```python
from build123d import *

# Parameters (mm, degrees)
F0_W          = 38
F0_H          = 23
F1_DEPTH      = 4.5
F2_T          = -2
F3_W          = 9
F3_H          = 2.5
F4_DEPTH      = 2
F5_W          = 2
F5_H          = 1
F6_DEPTH      = 2
F7_W          = 4
F7_H          = 4
F7_H_2        = 4.2236842105
F8_DEPTH      = 2
F9_DEPTH      = 0.5
F10_W         = 4
F10_H         = 4
F10_H_2       = 5.5396806626
F11_DEPTH     = 2
F12_DEPTH     = 0.5
F13_SIZE2     = 1
F13_SIZE      = 1
F14_T1_DEPTH  = 14.2867319519
F14_T3_DEPTH  = 14.2867319519
F14_T5_DEPTH  = 14.2867319519
F14_T10_DEPTH = 14.2867319519
F14_T15_DEPTH = 14.2867319519
F14_T20_DEPTH = 14.2867319519
F15_R         = 2
F10_H_3       = 1.5
F16_DEPTH     = 1
F7_H_3        = 1.5
F17_DEPTH     = 1
F18_SIZE2     = 0.99999
F18_SIZE      = 1.49999
F19_SIZE2     = 1.49999
F19_SIZE      = 0.99999
F20_SIZE2     = 0.99999
F20_SIZE      = 1.49999


# Not quite as in the source:
# - a fillet or chamfer that OpenCascade refuses, or shapes differently, is made with other operations: its cross-section is extruded or revolved along the edge and cut away or added
# - a fillet or chamfer is up to 0.001 mm smaller than in the source, because OpenCascade refuses the exact size


with BuildPart() as f1:
    # F0 (on Top) → F1 (new body)
    with BuildSketch(Plane.XY):
        Rectangle(F0_W, F0_H)
    extrude(amount=F1_DEPTH)

    # F2
    f2_openings = [f1.faces().sort_by_distance(p)[0] for p in [
        (0, 0, 4.5),
    ]]
    offset(amount=F2_T, openings=f2_openings)

    # F3 (on face) → F4 (cut, through all)
    with BuildSketch(Plane(origin=(-19, 0, 0), x_dir=(0, -1, 0), z_dir=(-1, 0, 0))):
        with Locations((0, 3.25)):
            Rectangle(F3_W, F3_H)
    extrude(amount=-F4_DEPTH, mode=Mode.SUBTRACT)

    # F5 (on face) → F6 (cut, through all)
    with BuildSketch(Plane(origin=(0, 11.5, 0), x_dir=(-1, 0, 0), z_dir=(0, 1, 0))):
        with Locations((-2.0402920675, 4)):
            Rectangle(F5_W, F5_H)
        with Locations((2.0402920675, 4)):
            Rectangle(F5_W, F5_H)
    extrude(amount=-F6_DEPTH, mode=Mode.SUBTRACT)

    # F7 (on face) → F8 (join)
    with BuildSketch(Plane(origin=(0, 11.5, 0), x_dir=(-1, 0, 0), z_dir=(0, 1, 0))):
        with Locations((-9.5, 8)):
            Rectangle(F7_W, F7_H)
        with Locations((-9.5, 3.8881578947)):
            Rectangle(F7_W, F7_H_2)
        with Locations((9.5, 8)):
            Rectangle(F7_W, F7_H)
        with Locations((9.5, 3.8881578947)):
            Rectangle(F7_W, F7_H_2)
    extrude(amount=F8_DEPTH)

    # F7 (on face) → F9 (join)
    with BuildSketch(Plane(origin=(0, 11.5, 0), x_dir=(-1, 0, 0), z_dir=(0, 1, 0))):
        with Locations((-9.5, 8)):
            Rectangle(F7_W, F7_H)
        with Locations((9.5, 8)):
            Rectangle(F7_W, F7_H)
    extrude(amount=-F9_DEPTH)

    # F10 (on face) → F11 (join)
    with BuildSketch(Plane.XZ.offset(11.5)):
        with Locations((0, 8)):
            Rectangle(F10_W, F10_H)
        with Locations((0, 3.2301596687)):
            Rectangle(F10_W, F10_H_2)
    extrude(amount=F11_DEPTH)

    # F10 (on face) → F12 (join)
    with BuildSketch(Plane.XZ.offset(11.5)):
        with Locations((0, 8)):
            Rectangle(F10_W, F10_H)
    extrude(amount=-F12_DEPTH)

    # F13
    f13_edges = [f1.edges().sort_by_distance(p)[0] for p in [
        (0, -11, 10),
        (-9.5, 11, 10),
        (9.5, 11, 10),
    ]]
    chamfer(f13_edges, length=F13_SIZE, length2=F13_SIZE2)

    # F14: chamfer of 2 on 6 edges, made by hand

    # F14_s2 → F14_t1 (cut)
    with BuildSketch(Plane.YZ.offset(2.3566340241)):
        Polygon((11.5, 10), (13.5, 8), (13.5, 10), align=None)
    extrude(amount=F14_T1_DEPTH, mode=Mode.SUBTRACT)

    # F14_s4 → F14_t3 (cut)
    with BuildSketch(Plane.YZ.offset(-16.6433659759)):
        Polygon((11.5, 10), (13.5, 8), (13.5, 10), align=None)
    extrude(amount=F14_T3_DEPTH, mode=Mode.SUBTRACT)

    # F14_s6 → F14_t5 (cut)
    with BuildSketch(Plane.YZ.offset(-7.1433659759)):
        Polygon((-11.5, 10), (-13.5, 8), (-13.5, 10), align=None)
    extrude(amount=F14_T5_DEPTH, mode=Mode.SUBTRACT)


with BuildPart() as f14_tool8:
    # F14_s9 → F14_t10 (new body)
    with BuildSketch(Plane.YZ.offset(-2.3566340241)):
        Polygon((11.5, 1.7763157895), (13.5, 3.7763157895), (13.5, 1.7763157895), align=None)
    extrude(amount=-F14_T10_DEPTH)

    split(bisect_by=Plane.XZ.offset(-11.5), keep=Keep.BOTTOM)


with BuildPart() as f1_1:
    add(f1.part)

    # F14_t7: cut F14_tool8
    add(f14_tool8.part, mode=Mode.SUBTRACT)


with BuildPart() as f14_tool13:
    # F14_s14 → F14_t15 (new body)
    with BuildSketch(Plane.YZ.offset(16.6433659759)):
        Polygon((13.5, 3.7763157895), (11.5, 1.7763157895), (13.5, 1.7763157895), align=None)
    extrude(amount=-F14_T15_DEPTH)

    split(bisect_by=Plane.XZ.offset(-11.5), keep=Keep.BOTTOM)


with BuildPart() as f1_2:
    add(f1_1.part)

    # F14_t12: cut F14_tool13
    add(f14_tool13.part, mode=Mode.SUBTRACT)


with BuildPart() as f14_tool18:
    # F14_s19 → F14_t20 (new body)
    with BuildSketch(Plane.YZ.offset(-7.1433659759)):
        Polygon((-11.5, 0.4603193374), (-13.5, 2.4603193374), (-13.5, 0.4603193374), align=None)
    extrude(amount=F14_T20_DEPTH)

    split(bisect_by=Plane.XZ.offset(11.5), keep=Keep.TOP)


with BuildPart() as f1_3:
    add(f1_2.part)

    # F14_t17: cut F14_tool18
    add(f14_tool18.part, mode=Mode.SUBTRACT)

    # F15
    f15_edges = [f1_3.edges().sort_by_distance(p)[0] for p in [
        (19, -11.5, 2.25),
        (19, 11.5, 2.25),
        (-19, 11.5, 2.25),
        (-19, -11.5, 2.25),
    ]]
    fillet(f15_edges, radius=F15_R)

    # F10 (on face) → F16 (cut)
    with BuildSketch(Plane.XZ.offset(11.5)):
        with Locations((0, 5.25)):
            Rectangle(F10_W, F10_H_3)
    extrude(amount=F16_DEPTH, mode=Mode.SUBTRACT)

    # F7 (on face) → F17 (cut)
    with BuildSketch(Plane(origin=(0, 11.5, 0), x_dir=(-1, 0, 0), z_dir=(0, 1, 0))):
        with Locations((9.5, 5.25)):
            Rectangle(F7_W, F7_H_3)
        with Locations((-9.5, 5.25)):
            Rectangle(F7_W, F7_H_3)
    extrude(amount=F17_DEPTH, mode=Mode.SUBTRACT)

    # F18 (size 1.5 and 1 in the source; OpenCascade refuses exactly that, so slightly less here)
    f18_edges = [f1_3.edges().sort_by_distance(p)[0] for p in [
        (0, -11, 6),
    ]]
    f18_side = f1_3.faces().sort_by_distance((0, -11.75, 6))[0]
    chamfer(f18_edges, length=F18_SIZE, length2=F18_SIZE2, reference=f18_side)

    # F19 (size 1 and 1.5 in the source; OpenCascade refuses exactly that, so slightly less here)
    f19_edges = [f1_3.edges().sort_by_distance(p)[0] for p in [
        (-9.5, 11, 6),
    ]]
    f19_side = f1_3.faces().sort_by_distance((-9.5, 11, 7.5))[0]
    chamfer(f19_edges, length=F19_SIZE, length2=F19_SIZE2, reference=f19_side)

    # F20 (size 1.5 and 1 in the source; OpenCascade refuses exactly that, so slightly less here)
    f20_edges = [f1_3.edges().sort_by_distance(p)[0] for p in [
        (9.5, 11, 6),
    ]]
    f20_side = f1_3.faces().sort_by_distance((9.5, 11.75, 6))[0]
    chamfer(f20_edges, length=F20_SIZE, length2=F20_SIZE2, reference=f20_side)


solid = f1_3.part
```
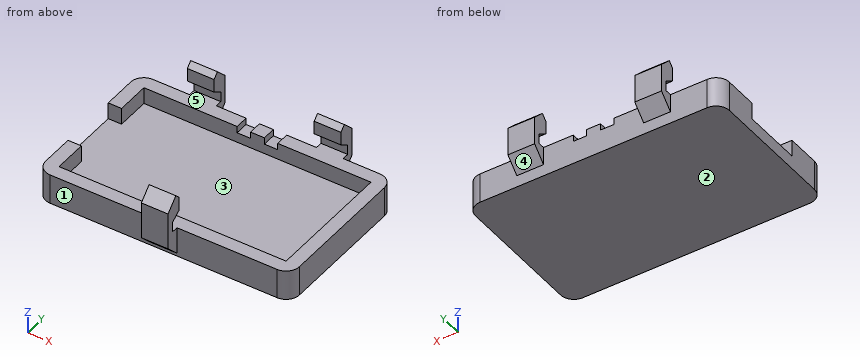
Here's how the part is built. I have some questions about the finished solid (model axes, mm). Face numbers are marked on the shaded views. A direction names the side the tool comes from. Coordinates: 2 decimals unless noted, no trailing zeros. Write each loop counter-clockwise with the first axis right and the second up, starting at its lowest first coordinate (ties: lowest second). Pieces come first, ordered by that corner, then holes. Notation, with made-up numbers: (32.5, -37.5) - (50.5, -37.5) arc R31 cw to (50.5, -4.5) - close; hole circle Ø4 at (-8.75, 73.25). An arc over 180 degrees is marked (long way). One line per item, written item: value.
1) Suppose I cut it at A-A on x = -15.5. Write out the boundary of the cut face in (y, z).
Model answer:
outline: (-11.5, 0) - (11.5, 0) - (11.5, 4.5) - (9.5, 4.5) - (9.5, 2) - (-9.5, 2) - (-9.5, 4.5) - (-11.5, 4.5) - close
2) On a 3-axis mill with a long thin cutter (end or side, diameter ignored), from which of +Z, -Z, +X, -X, +Y, -Y can I reach the whole of each face in a straight line? I mean the marked faces 4 and 5. Say none if no direction works.
Model answer:
face 4: -Z, +X, -X, +Y
face 5: +X, -X, -Y
3) We'd pull the mould along Y, two halves only. Please class the marked faces 1, 2 and 3: pulls with the +Y half, pulls with the -Y half, needs draft (parallel to the pull), parting line crosses it, or undercut.
Model answer:
face 1: pulls with the -Y half
face 2: needs draft
face 3: undercut
4) I'm going to push flat-ended pins straight in: P1, Ø0.8, axis at x = -9, z = 5, coming from the -Y side; P2, Ø1.6, axis at x = -0.5, y = 10.5, coming from the +Z side; P3, Ø1.6, axis at x = 8.5, z = 5, coming from the -Y side. Where does each tip first touch, or does it pass through?
Model answer:
P1: stops at y = 12.5
P2: stops at z = 4.5
P3: stops at y = -11.5
5) I need wall thicknesses on line 1 along X through (y, z) = (-5.5, 3.75); line 2 along Y through (x, z) = (-13, 0.5); line 3 along Z through (x, y) = (-13, -8). Which ranges of each line are inside material? Lowest first, please.
Model answer:
line 1: x = -19 to -17, 17 to 19
line 2: y = -11.5 to 11.5
line 3: z = 0 to 2
6) Suppose I cut it at D-D on y = 0. Write out the boundary of the cut face in (x, z), and give its area (3 significant figures).
Model answer:
outline: (-19, 0) - (19, 0) - (19, 4.5) - (17, 4.5) - (17, 2) - (-19, 2) - close
area: 81.0 mm²
7) Suppose I cut it at B-B on y = 6. Write out the boundary of the cut face in (x, z).
Model answer:
outline: (-19, 0) - (19, 0) - (19, 4.5) - (17, 4.5) - (17, 2) - (-17, 2) - (-17, 4.5) - (-19, 4.5) - close
